The listing builds one solid part. Answer for the finished solid, in the listing's coordinates (mm). A direction names the side the tool comes from. Round coordinates to 2 decimals unless told otherwise and drop trailing zeros. Loops run counter-clockwise (first coordinate to the right, second up) from the corner with the lowest first, then second, coordinate; pieces in that order, holes last. Notation, with made-up numbers: M 58.25,13 L 102.25,13 A36 cw 102.25,50 Z; hole C 72.5,36 d8. An arc over 180 degrees is marked long. Answer as a JSON object with one key per item and string values.
```python
from build123d import *

# Parameters (mm, degrees)
CROQUIS1_W               = 208
CROQUIS1_H               = 147
SALIENTE_EXTRUIR1_DEPTH  = 5
CORTAR_EXTRUIR1_DEPTH    = 128.449009412
SIMETR_A2_COPY_1_DEPTH   = 128.449009412
REDONDEO1_R              = 10
SALIENTE_EXTRUIR3_DEPTH  = 20
REDONDEO2_R              = 5
REDONDEO2_OF_SIMETR_A3_R = 5
SIMETR_A4_START          = -20
SIMETR_A4_DEPTH          = 20
ESCALA1_SCALE            = 2


# Read off the part's stored shape, not the designer's step: Simetría4
with BuildPart() as part:
    # Croquis1 → Saliente-Extruir1 (new body)
    with BuildSketch(Plane(origin=(0, 0, 0), x_dir=(1, 0, 0), z_dir=(0, 1, 0))):
        Rectangle(CROQUIS1_W, CROQUIS1_H)
    extrude(amount=SALIENTE_EXTRUIR1_DEPTH)

    # Croquis3 → Cortar-Extruir1 (cut, through all)
    with BuildSketch(Plane(origin=(0, 5, 0), x_dir=(1, 0, 0), z_dir=(0, 1, 0))):
        with BuildLine():
            Line((-89, 80.855395091), (-89, 60.855395091))
            Line((-89, 60.855395091), (-44, 60.855395091))
            Line((-44, 60.855395091), (-44, 55.855395091))
            Line((-44, 55.855395091), (-29, 55.855395091))
            Line((-29, 55.855395091), (-29, 60.855395091))
            Line((-29, 60.855395091), (-14, 60.855395091))
            ThreePointArc((-14, 60.855395091), (-6.928932188, 61.357920408), (0, 62.855395091))
            Line((0, 62.855395091), (0, 82.855395091))
            Line((0, 82.855395091), (-89, 82.855395091))
            Line((-89, 82.855395091), (-89, 80.855395091))
        make_face()
    cortar_extruir1 = extrude(amount=-CORTAR_EXTRUIR1_DEPTH, mode=Mode.SUBTRACT)

    # Simetría1: Cortar-Extruir1 across plane
    add(cortar_extruir1.mirror(Plane.XY), mode=Mode.SUBTRACT)

    # Simetría2: Cortar-Extruir1 across plane
    add(cortar_extruir1.mirror(Plane(origin=(0, 0, 0), x_dir=(0, 0, 1), z_dir=(1, 0, 0))), mode=Mode.SUBTRACT)

    # Simetría2 copy 1 sketch → Simetría2 copy 1 (cut, through all)
    with BuildSketch(Plane(origin=(0, 5, 0), x_dir=(-1, 0, 0), z_dir=(0, 1, 0))):
        with BuildLine():
            Line((-89, 80.855395091), (-89, 60.855395091))
            Line((-89, 60.855395091), (-44, 60.855395091))
            Line((-44, 60.855395091), (-44, 55.855395091))
            Line((-44, 55.855395091), (-29, 55.855395091))
            Line((-29, 55.855395091), (-29, 60.855395091))
            Line((-29, 60.855395091), (-14, 60.855395091))
            ThreePointArc((-14, 60.855395091), (-6.928932188, 61.357920408), (0, 62.855395091))
            Line((0, 62.855395091), (0, 82.855395091))
            Line((0, 82.855395091), (-89, 82.855395091))
            Line((-89, 82.855395091), (-89, 80.855395091))
        make_face()
    extrude(amount=-SIMETR_A2_COPY_1_DEPTH, mode=Mode.SUBTRACT)

    # Redondeo1
    redondeo1_edges = [part.edges().sort_by_distance(p)[0] for p in [
        (-104, 2.5, -73.5),
        (104, 2.5, -73.5),
        (104, 2.5, 73.5),
        (-104, 2.5, 73.5),
    ]]
    fillet(redondeo1_edges, radius=REDONDEO1_R)

    # Croquis5 → Saliente-Extruir3 (add)
    with BuildSketch(Plane.XZ):
        Polygon((-104, 37.458190843), (-11, 37.458190843), (-11, 60.945476237), (-14, 60.855395091), (-14, 40.458190843), (-104, 40.458190843), align=None)
    saliente_extruir3 = extrude(amount=SALIENTE_EXTRUIR3_DEPTH)

    # Redondeo2
    redondeo2_edges = [part.edges().sort_by_distance(p)[0] for p in [
        (-11, -10, 37.458190843),
    ]]
    fillet(redondeo2_edges, radius=REDONDEO2_R)

    # Simetría3: Saliente-Extruir3 across plane
    add(saliente_extruir3.mirror(Plane.XY))

    # Redondeo2 of Simetría3
    redondeo2_of_simetr_a3_edges = [part.edges().sort_by_distance(p)[0] for p in [
        (-11, -10, -37.458190843),
    ]]
    fillet(redondeo2_of_simetr_a3_edges, radius=REDONDEO2_OF_SIMETR_A3_R)

    # Simetría4 outline → Simetría4 (add)
    with BuildSketch(Plane(origin=(0, 0, 0), x_dir=(1, 0, 0), z_dir=(0, 1, 0)).offset(SIMETR_A4_START)):
        with BuildLine():
            Line((104, -40.458190843), (104, -37.458190843))
            Line((104, -37.458190843), (16, -37.458190843))
            ThreePointArc((16, -37.458190843), (12.464466094, -38.922656937), (11, -42.458190843))
            Line((11, -42.458190843), (11, -60.945476237))
            Line((11, -60.945476237), (14, -60.855395091))
            Line((14, -60.855395091), (14, -40.458190843))
            Line((14, -40.458190843), (104, -40.458190843))
        make_face()
        with BuildLine():
            Line((104, 37.458190843), (104, 40.458190843))
            Line((104, 40.458190843), (14, 40.458190843))
            Line((14, 40.458190843), (14, 60.855395091))
            Line((14, 60.855395091), (11, 60.945476237))
            Line((11, 60.945476237), (11, 42.458190843))
            ThreePointArc((11, 42.458190843), (12.464466094, 38.922656937), (16, 37.458190843))
            Line((16, 37.458190843), (104, 37.458190843))
        make_face()
    extrude(amount=SIMETR_A4_DEPTH)


with BuildPart() as part_1:
    # Escala1: scaled about (0, 0.344872769, 0)
    add(part.part.scale(ESCALA1_SCALE).moved(Location((0, -0.344872769, 0))))


solid = part_1.part
```
Item 1: Flat-ended cylindrical pins translate along their axes: P1, Ø20, axis at x = -89.5, z = 107, coming from the -Y side; P2, Ø4, axis at y = -8.5, z = 89.5, coming from the -X side; P3, Ø1, axis at x = -82.5, y = -18, coming from the -Z side. Find the tip coordinate at first contact, or state that the pin passes through.
Values follow:
{"P1": "y = -0.34", "P2": "x = -28", "P3": "z = -80.92"}
Item 2: The part is cut by section B-B (x = -64). Give the vertices of the cut face in (y, z), then the cut area to 3 significant figures.
Values follow:
{"outline": "M -40.34,-80.92 L -0.34,-80.92 L -0.34,-111.71 L 9.66,-111.71 L 9.66,111.71 L -0.34,111.71 L -0.34,80.92 L -40.34,80.92 L -40.34,74.92 L -0.34,74.92 L -0.34,-74.92 L -40.34,-74.92 Z", "area": "2,710 mm^2"}
Item 3: Straight lines are drawn through the part: line 1 (Z direction, x = 165.5, y = -8.5); line 2 (X direction, y = -34, z = 86); line 3 (Y direction, x = -81, z = 97.5). For each, find the intervals that lie inside material, in ascending order.
Values follow:
{"line 1": "-80.92 to -74.92, 74.92 to 80.92", "line 2": "-28 to -22, 22 to 28", "line 3": "-0.34 to 9.66"}
Item 4: The part is cut by section D-D (x = -109). Give the vertices of the cut face in (y, z).
Values follow:
{"outline": "M -40.34,-80.92 L -0.34,-80.92 L -0.34,-121.71 L 9.66,-121.71 L 9.66,121.71 L -0.34,121.71 L -0.34,80.92 L -40.34,80.92 L -40.34,74.92 L -0.34,74.92 L -0.34,-74.92 L -40.34,-74.92 Z"}
Item 5: The part is cut by section C-C (z = 11). Give the vertices of the cut face in (x, y), then the cut area to 3 significant figures.
Values follow:
{"outline": "M -208,-0.34 L 208,-0.34 L 208,9.66 L -208,9.66 Z", "area": "4,160 mm^2"}
Item 6: Which of the six approach directions +Z, -Z, +X, -X, +Y, -Y give full straight-line access (tool end or side, diameter ignored) to faces 1 (the face through (-28, -20, 102)), 2 (the face through (43, 5, 121.711)), 3 (the face through (22, -21, -104)), 4 (the face through (119, -21, -80.916)), 5 (the face through (-73, 5, -111.711))?
Values follow:
{"face 1": "+Z, -X, -Y", "face 2": "+Z, +Y, -Y", "face 3": "+Z, -Z, -Y", "face 4": "-Z, +X, -Y", "face 5": "-Z, +Y, -Y"}
Item 7: Determine the mould class of faces 6 (the face through (183, 5, -147)), 7 (the face through (-28, -20, -102)), 8 (the face through (134, 5, -121.711)) for opening direction X: released by +X, released by -X, zero draft, split by the parting line, or undercut.
Values follow:
{"face 6": "zero draft", "face 7": "released by -X", "face 8": "undercut"}
Item 8: The part is cut by section A-A (y = -32). Give the vertices of the cut face in (x, z).
Values follow:
{"outline": "M -208,-80.92 L -28,-80.92 L -28,-121.71 L -22,-121.89 L -22,-84.92 A10 ccw -32,-74.92 L -208,-74.92 Z; M -208,74.92 L -32,74.92 A10 ccw -22,84.92 L -22,121.89 L -28,121.71 L -28,80.92 L -208,80.92 Z; M 22,-121.89 L 28,-121.71 L 28,-80.92 L 208,-80.92 L 208,-74.92 L 32,-74.92 A10 ccw 22,-84.92 Z; M 22,84.92 A10 ccw 32,74.92 L 208,74.92 L 208,80.92 L 28,80.92 L 28,121.71 L 22,121.89 Z"}
